```python
from build123d import *

# Parameters (mm, degrees)
SKETCH_1_W               = 14.5
SKETCH_1_H               = 14.5
EXTRUDE_1_DEPTH          = 10.5
SKETCH_4_R               = 2.15
CUT_EXTRUDE_2_DEPTH      = 8.25
CUT_EXTRUDE_2_DEPTH_BACK = 8.25
SKETCH_6_W               = 14.5
SKETCH_6_H               = 14.5
EXTRUDE_2_DEPTH          = 13.5
SKETCH_9_W               = 4
SKETCH_9_H               = 24
EXTRUDE_3_DEPTH          = 12
SKETCH_10_W              = 5.6
SKETCH_10_H              = 24
EXTRUDE_4_DEPTH          = 1
SKETCH_11_R              = 4.5
CUT_EXTRUDE_3_DEPTH      = 7.85
SKETCH_12_R              = 1.9
CUT_EXTRUDE_4_DEPTH      = 1
CUT_EXTRUDE_4_DEPTH_BACK = 16.5
FILLET_1_R               = 4
FILLET_3_R               = 1


with BuildPart() as part:
    # 草图1 → 凸台-拉伸1 (new body)
    with BuildSketch(Plane(origin=(0, 0, 0), x_dir=(1, 0, 0), z_dir=(0, 1, 0))):
        Rectangle(SKETCH_1_W, SKETCH_1_H)
        with BuildLine():
            Line((3.465905365, -3.1), (-3.465905365, -3.1))
            ThreePointArc((-3.465905365, -3.1), (-4.65, 0), (-3.465905365, 3.1))
            Line((-3.465905365, 3.1), (3.465905365, 3.1))
            ThreePointArc((3.465905365, 3.1), (4.65, 0), (3.465905365, -3.1))
        make_face(mode=Mode.SUBTRACT)
    extrude(amount=EXTRUDE_1_DEPTH)

    # 草图4 → 切除-拉伸2 (cut, two sides)
    with BuildSketch(Plane.XY) as cut_extrude_2_sk:
        with Locations((0, 4)):
            Circle(SKETCH_4_R)
    extrude(amount=CUT_EXTRUDE_2_DEPTH, mode=Mode.SUBTRACT)
    extrude(cut_extrude_2_sk.sketch, amount=-CUT_EXTRUDE_2_DEPTH_BACK, mode=Mode.SUBTRACT)

    # 草图6 → 凸台-拉伸2 (add)
    with BuildSketch(Plane.XZ):
        Rectangle(SKETCH_6_W, SKETCH_6_H)
        with BuildLine():
            Line((-3.465905365, -3.1), (3.465905365, -3.1))
            ThreePointArc((3.465905365, -3.1), (4.65, 0), (3.465905365, 3.1))
            Line((3.465905365, 3.1), (-3.465905365, 3.1))
            ThreePointArc((-3.465905365, 3.1), (-4.65, 0), (-3.465905365, -3.1))
        make_face(mode=Mode.SUBTRACT)
    extrude(amount=EXTRUDE_2_DEPTH)

    # 草图9 → 凸台-拉伸3 (add)
    with BuildSketch(Plane.XY.offset(-3.1)):
        with Locations((5.25, -1.5)):
            Rectangle(SKETCH_9_W, SKETCH_9_H)
    extrude_3 = extrude(amount=-EXTRUDE_3_DEPTH)

    # 镜向1: 凸台-拉伸3 across plane
    add(extrude_3.mirror(Plane.XY))

    # 草图10 → 凸台-拉伸4 (add)
    with BuildSketch(Plane(origin=(7.25, 0, 0), x_dir=(0, 0, -1), z_dir=(1, 0, 0))):
        with Locations((-12.3, -1.5)):
            Rectangle(SKETCH_10_W, SKETCH_10_H)
        with Locations((12.3, -1.5)):
            Rectangle(SKETCH_10_W, SKETCH_10_H)
    extrude(amount=EXTRUDE_4_DEPTH)

    # 草图11 → 切除-拉伸3 (cut)
    with BuildSketch(Plane.XY.offset(15.1)):
        with Locations((0, 4)):
            Circle(SKETCH_11_R)
    cut_extrude_3 = extrude(amount=-CUT_EXTRUDE_3_DEPTH, mode=Mode.SUBTRACT)

    # 镜向2: 切除-拉伸3 across plane
    add(cut_extrude_3.mirror(Plane.XY), mode=Mode.SUBTRACT)

    # 草图12 → 切除-拉伸4 (cut, two sides)
    with BuildSketch(Plane(origin=(8.25, 0, 0), x_dir=(0, 0, -1), z_dir=(1, 0, 0))) as cut_extrude_4_sk:
        with Locations((12, -1.5)):
            Circle(SKETCH_12_R)
        with Locations((-12, -1.5)):
            Circle(SKETCH_12_R)
    extrude(amount=CUT_EXTRUDE_4_DEPTH, mode=Mode.SUBTRACT)
    extrude(cut_extrude_4_sk.sketch, amount=-CUT_EXTRUDE_4_DEPTH_BACK, mode=Mode.SUBTRACT)

    # 圆角1
    fillet_1_edges = [part.edges().sort_by_distance(p)[0] for p in [
        (-7.25, -1.5, 7.25),
        (-7.25, -1.5, -7.25),
    ]]
    fillet(fillet_1_edges, radius=FILLET_1_R)

    # 圆角3
    fillet_3_edges = [part.edges().sort_by_distance(p)[0] for p in [
        (3.25, -6.30623745, 15.1),
        (3.25, -6.30623745, -15.1),
        (3.25, 8.80623745, -15.1),
        (3.25, 8.80623745, 15.1),
    ]]
    fillet(fillet_3_edges, radius=FILLET_3_R)


solid = part.part
```
Design review of the part built by this model. Coordinates are the model's own, in mm. A direction names the side the tool comes from. Give positions to 0.01 mm unless a question says otherwise; leave off trailing zeros. Order: outer loops, then holes, each group sorted by start corner. A loop starts at its lowest first (then second) coordinate and runs counter-clockwise, first axis right, second up. Notation, with made-up numbers: (51, -24.75) -> (73, -24.75) arc R26 ccw to (73, -4.75) -> close; hole circle Ø2 at (15, 84.5). An arc over 180 degrees is marked (long way). Write item = value, one per line. Start each with the question number.
(1) We need section A-A on y = -1.5. Write out the cut boundary in (x, z), plus the area to 3 significant figures.
(2) We need section C-C on x = -2.75. Write out the cut boundary in (y, z).
(3) For pin 1 (1.5 mm diameter, centred on x = -2, y = 1, fed in from -Z); pin 2 (7.5 mm diameter, centred on x = -1.5, y = -4.5, fed in from +Z); pin 3 (3.5 mm diameter, centred on y = -3.5, z = 12, fed in from -X); pin 4 (2 mm diameter, centred on x = 1, z = 9, fed in from -Y), all flat-tipped, find the tip position at first contact; note any pin that passes through.
(4) We need section B-B on z = -12. Write out the cut boundary in (x, y), plus the area to 3 significant figures.
(5) For faces 4 (the face through (0, -1, -3.1)), 5 (the face through (8, -2, -9.5)), 6 (the face through (4.5, 4, 11.2)), 7 (the face through (3.25, -6, -11)), list the 3-axis set-ups (+Z, -Z, +X, -X, +Y, -Y) from which the entire face can be reached by the end or side of a thin tool; tool diameter is ignored.
(6) We need section D-D on y = 4. Write out the cut boundary in (x, z), plus the area to 3 significant figures.
(7) To check wall thickness, follow line 1 along Y through (x, z) = (0, -6.3); line 2 along Y through (x, z) = (4.65, -12); line 3 along Z through (x, y) = (-1, -1). State the ranges of each line that lie inside material, in increasing order.
(8) Mouldability with a two-part tool opening along Y and no side actions: class faces 1 (the face through (2, 10.5, 4)), 2 (the face through (-6.109, -1.332, 6.047)), 3 (the face through (5.785, -2.228, -13.755)) as +Y half, -Y half, draft (parallel to the pull), parting line (faces both ways), or undercut.
Numbers:
q1.outline = (-7.25, -3.25) arc R4 ccw to (-3.25, -7.25) -> (3.25, -7.25) -> (3.25, -10.1) -> (8.25, -10.1) -> (8.25, -9.5) -> (7.25, -9.5) -> (7.25, 9.5) -> (8.25, 9.5) -> (8.25, 10.1) -> (3.25, 10.1) -> (3.25, 7.25) -> (-3.25, 7.25) arc R4 ccw to (-7.25, 3.25) -> close; (3.25, -14.1) arc R1 ccw to (4.25, -15.1) -> (8.25, -15.1) -> (8.25, -13.9) -> (3.25, -13.9) -> close; (3.25, 13.9) -> (8.25, 13.9) -> (8.25, 15.1) -> (4.25, 15.1) arc R1 ccw to (3.25, 14.1) -> close; hole (-3.47, -3.1) -> (3.47, -3.1) arc R4.65 ccw to (3.47, 3.1) -> (-3.47, 3.1) arc R4.65 ccw to start
q1.area = 186 mm^2
q2.outline = (-13.5, -7.25) -> (10.5, -7.25) -> (10.5, -3.1) -> (-13.5, -3.1) -> close; (-13.5, 3.1) -> (10.5, 3.1) -> (10.5, 7.25) -> (-13.5, 7.25) -> close
q3.pin_1 = -7.25
q3.pin_2 = 7.25
q3.pin_3 = 3.25
q3.pin_4 = through
q4.outline = (3.25, -13.5) -> (8.25, -13.5) -> (8.25, -3.4) -> (3.25, -3.4) -> close; (3.25, 0.4) -> (8.25, 0.4) -> (8.25, 10.5) -> (3.25, 10.5) -> (3.25, 7.11) arc R4.5 cw to (3.25, 0.89) -> close
q4.area = 95.6 mm^2
q5.face_4 = +Y, -Y
q5.face_5 = +X, +Y, -Y
q5.face_6 = +Z, -X
q5.face_7 = -Z, -X, +Y, -Y
q6.outline = (-7.25, -3.25) arc R4 ccw to (-3.25, -7.25) -> (-2.15, -7.25) -> (-2.15, -3.1) -> (-3.47, -3.1) arc R4.65 cw to (-3.47, 3.1) -> (-2.15, 3.1) -> (-2.15, 7.25) -> (-3.25, 7.25) arc R4 ccw to (-7.25, 3.25) -> close; (2.15, -7.25) -> (4.5, -7.25) -> (4.5, -15.1) -> (8.25, -15.1) -> (8.25, -9.5) -> (7.25, -9.5) -> (7.25, 9.5) -> (8.25, 9.5) -> (8.25, 15.1) -> (4.5, 15.1) -> (4.5, 7.25) -> (2.15, 7.25) -> (2.15, 3.1) -> (3.47, 3.1) arc R4.65 cw to (3.47, -3.1) -> (2.15, -3.1) -> close
q6.area = 169 mm^2
q7.line_1 = -13.5 to 1.85, 6.15 to 10.5
q7.line_2 = -13.5 to -3.4, 0.4 to 10.5
q7.line_3 = -7.25 to -3.1, 3.1 to 7.25
q8.face_1 = +Y half
q8.face_2 = draft
q8.face_3 = undercut
